Here's how the part is built. I have some questions about the finished solid (model axes, mm). A direction names the side the tool comes from. Round coordinates to 2 decimals unless told otherwise and drop trailing zeros. Write each loop counter-clockwise with the first axis right and the second up, starting at its lowest first coordinate (ties: lowest second). Pieces come first, ordered by that corner, then holes. Notation, with made-up numbers: (12.25, 63) - (39.25, 63) arc R20 cw to (39.25, 100) - close; hole circle Ø8 at (8.25, -24). An arc over 180 degrees is marked (long way). One line per item, written item: value. Start each with the question number.
Item 1: Imagine slicing it at C-C, the plane y = 38. Please give me the cut outline in (x, z).
Item 2: Thinking about a two-plate mould opening in Y: for faces 1 (the face through (138, 0, -16)), 2 (the face through (-7.098, 1.002, -8.294)), 3 (the face through (138, 28, 0)), which applies, released by +Y, released by -Y, zero draft, split by the parting line, or undercut?
Item 3: For faces 4 (the face through (138, 2.032, -15)), 5 (the face through (-7.098, 1.002, -20.994)), which set-ups out of +Z, -Z, +X, -X, +Y, -Y let a thin tool reach every point of the face, with its end or its side?
Item 4: Imagine slicing it at A-A, the plane z = -4.5. Please give me the cut outline in (x, y), then the cut area to 3 significant figures.
Item 5: Imagine slicing it at B-B, the plane x = 215.5. Please give me the cut outline in (y, z), then the cut area to 3 significant figures.
Item 6: If I drill on line 1 (Z direction, x = -6.35, y = 53.6); line 2 (Y direction, x = 84.5, z = -27); line 3 (Z direction, x = 21.5, y = 47.5), over which ranges is the centre line in solid material (lowest first)?
Item 7: For P1, Ø12, axis at y = 43, z = -17, coming from the -X side; P2, Ø12, axis at x = 62.5, y = 35, coming from the -Z side; P3, Ø1.7, axis at y = 39, z = 0.5, coming from the -X side; P4, Ø0.6, axis at x = 284, y = 53.5, coming from the +Z side, each with a flat end and sliding along its axis, tell me the tip position at first contact or that it passes through.
Autodesk Inventor part; units mm, degrees
ref_plane "YZ Plane" through (0, 0, 0) normal (1, 0, 0) x (0, 1, 0)
ref_plane "XZ Plane" through (0, 0, 0) normal (0, 1, 0) x (-1, 0, 0)
ref_plane "XY Plane" through (0, 0, 0) normal (0, 0, 1) x (1, 0, 0)
sketch "Sketch1" plane through (0, 0, 0) normal (0, 0, 1) x (1, 0, 0)
  line L0 (0, 0) -> (279.4, 0)
  line L1 (279.4, 0) -> (279.4, 54.864)
  line L2 (279.4, 54.864) -> (0, 54.864)
  line L3 (0, 54.864) -> (0, 0)
  dimension "d0" = 54.864
  dimension "d1" = 279.4
extrude "Plate1" add sketch "Sketch1" along normal blind 2.032
sketch "Sketch2" plane through (279.4, 52.832, 2.032) normal (0, 1, 0) x (-1, 0, 0)
  line L0 (279.4, 0) -> (0, 0)
  line L1 (0, 0) -> (0, -31.75)
  line L2 (0, -31.75) -> (279.4, -31.75)
  line L3 (279.4, -31.75) -> (279.4, 0)
edge flange "Flange1" height 31.75 angle 90 thickness 2.032 bend radius 1.27 thickness toward (0, 1, 0) relief tear relief width 2.032 relief depth 1.016 edges at (139.7, 54.864, 0) wall of the first edge with corners at (0, 52.832, 2.032) (279.4, 52.832, 2.032) (279.4, 52.832, -29.718) (0, 52.832, -29.718)
bend "Bend1"
corner "Corner1"
sketch "Sketch3" plane through (0, 2.032, 2.032) normal (0, -1, 0) x (1, 0, 0)
  line L0 (279.4, 0) -> (0, 0)
  line L1 (0, 0) -> (0, -31.75)
  line L2 (0, -31.75) -> (279.4, -31.75)
  line L3 (279.4, -31.75) -> (279.4, 0)
edge flange "Flange2" height 31.75 angle 90 thickness 2.032 bend radius 1.27 thickness toward (0, -1, 0) relief tear relief width 2.032 relief depth 1.016 edges at (139.7, 0, 0) wall of the first edge with corners at (279.4, 2.032, 2.032) (0, 2.032, 2.032) (0, 2.032, -29.718) (279.4, 2.032, -29.718)
bend "Bend2"
corner "Corner2"
sketch "Sketch4" plane through (279.4, 52.832, -29.718) normal (1, 0, 0) x (0, 0, -1)
  line L0 (-28.448, 2.032) -> (-28.448, 0)
  line L1 (-28.448, 0) -> (0, 0)
  line L2 (0, 0) -> (0, 2.032)
  line L3 (0, 2.032) -> (-28.448, 2.032)
  arc A0 (-28.448, 2.032) -> (-31.75, -1.27) centre (-28.448, -1.27) ccw
  line L4 (-29.718, -1.27) -> (-31.75, -1.27)
  arc A1 (-28.448, 0) -> (-29.718, -1.27) centre (-28.448, -1.27) ccw
  line L5 (-28.448, -50.8) -> (-28.448, -52.832)
  line L6 (-28.448, -52.832) -> (0, -52.832)
  line L7 (0, -50.8) -> (0, -52.832)
  line L8 (-28.448, -50.8) -> (0, -50.8)
  arc A2 (-29.718, -49.53) -> (-28.448, -50.8) centre (-28.448, -49.53) ccw
  line L9 (-31.75, -49.53) -> (-29.718, -49.53)
  arc A3 (-31.75, -49.53) -> (-28.448, -52.832) centre (-28.448, -49.53) ccw
  point P0 (-29.718, -52.832)
extrude "Extrusion1" add sketch "Sketch4" along normal blind 12.7 contours L3 L2 L1 L0 | L8 L7 L6 L5
sketch "Sketch5" plane through (0, 52.832, -29.718) normal (-1, 0, 0) x (0, 0, 1)
  line L0 (28.448, 0) -> (28.448, 2.032)
  line L1 (28.448, 2.032) -> (0, 2.032)
  line L2 (0, 0) -> (0, 2.032)
  line L3 (28.448, 0) -> (0, 0)
  arc A0 (29.718, -1.27) -> (28.448, 0) centre (28.448, -1.27) ccw
  line L4 (31.75, -1.27) -> (29.718, -1.27)
  arc A1 (31.75, -1.27) -> (28.448, 2.032) centre (28.448, -1.27) ccw
  line L5 (28.448, -52.832) -> (28.448, -50.8)
  line L6 (28.448, -50.8) -> (0, -50.8)
  line L7 (0, -50.8) -> (0, -52.832)
  line L8 (0, -52.832) -> (28.448, -52.832)
  arc A2 (28.448, -52.832) -> (31.75, -49.53) centre (28.448, -49.53) ccw
  line L9 (29.718, -49.53) -> (31.75, -49.53)
  arc A3 (28.448, -50.8) -> (29.718, -49.53) centre (28.448, -49.53) ccw
  point P0 (29.718, -52.832)
extrude "Extrusion2" add sketch "Sketch5" along normal blind 12.7 contours L3 L2 L1 L0 | L8 L7 L6 L5
sketch "Sketch6" plane through (279.4, 54.864, -1.27) normal (0, 1, 0) x (1, 0, 0)
  line L0 (0, -3.302) -> (-279.4, -3.302)
  line L1 (12.7, 28.448) -> (12.7, 0)
  line L2 (-292.1, 0) -> (-292.1, 28.448)
  point P0 (-279.4, -1.27)
  point P1 (6.35, 9.398)
  point P2 (6.35, 22.098)
  point P3 (-285.75, 9.398)
  point P4 (-285.75, 22.098)
  dimension "d27" = 12.7
  dimension "d28" = 12.7
  dimension "d29" = 6.35
  dimension "d30" = 6.35
hole "Hole1" at (285.75, 54.864, -10.668) at (285.75, 54.864, -23.368) at (-6.35, 54.864, -10.668) at (-6.35, 54.864, -23.368) direction (0, -1, 0) diameter 4.9784 end through all
equation "\"d36\" = Thickness"
equation "\"d2\" = Thickness"
equation "\"d3\" = BendReliefWidth"
equation "\"d4\" = BendReliefDepth"
equation "\"d5\" = MinimumRemnant"
equation "\"d6\" = TransitionRadius"
equation "\"d9\" = BendRadius"
equation "\"d10\" = CornerReliefSize"
equation "\"d11\" = GapSize"
equation "\"d12\" = JacobiRadiusSize"
equation "\"d13\" = BendReliefWidth"
equation "\"d14\" = BendReliefDepth"
equation "\"d15\" = MinimumRemnant"
equation "\"d16\" = TransitionRadius"
equation "\"d19\" = BendRadius"
equation "\"d20\" = CornerReliefSize"
equation "\"d21\" = GapSize"
equation "\"d22\" = JacobiRadiusSize"
equation "\"BendReliefWidth\" = Thickness"
equation "\"BendReliefDepth\" = 0.5 * Thickness"
equation "\"CornerReliefSize\" = 4 * Thickness"
equation "\"MinimumRemnant\" = 2 * Thickness"
equation "\"TransitionRadius\" = BendRadius"
equation "\"JacobiRadiusSize\" = BendRadius"
equation "\"GapSize\" = Thickness"
properties part number "Back brace" material "Aluminum 6061"
Values follow:
1. outline: (0, 0) - (279.4, 0) - (279.4, 2.03) - (0, 2.03) - close
2. face 1: released by -Y
2. face 2: zero draft
2. face 3: undercut
3. face 4: -Z, +X, -X
3. face 5: +Y, -Y
4. outline: (-12.7, 0) - (292.1, 0) - (292.1, 2.03) - (-12.7, 2.03) - close; (-12.7, 52.83) - (292.1, 52.83) - (292.1, 54.86) - (-12.7, 54.86) - close
4. area: 1,240 mm^2
5. outline: (0, -29.72) - (2.03, -29.72) - (2.03, -1.27) arc R1.27 cw to (3.3, 0) - (51.56, 0) arc R1.27 cw to (52.83, -1.27) - (52.83, -29.72) - (54.86, -29.72) - (54.86, -1.27) arc R3.3 ccw to (51.56, 2.03) - (3.3, 2.03) arc R3.3 ccw to (0, -1.27) - close
5. area: 228 mm^2
6. line 1: z = -29.72 to -25.86, -20.88 to -13.16, -8.18 to -1.27
6. line 2: y = 0 to 2.03, 52.83 to 54.86
6. line 3: z = 0 to 2.03
7. P1: passes through
7. P2: stops at z = 0
7. P3: stops at x = 0
7. P4: stops at z = -1.27
